Geometry check sheet. Reference: the model listing, model coordinates, mm. Coordinates: 2 decimals unless noted, no trailing zeros. Write each loop counter-clockwise with the first axis right and the second up, starting at its lowest first coordinate (ties: lowest second). Pieces come first, ordered by that corner, then holes. Notation, with made-up numbers: (36, -13.5) -> (80, -13.5) arc R38 cw to (80, 25.5) -> close; hole circle Ø3 at (-1, -25.75). An arc over 180 degrees is marked (long way). Answer as CSV lines item,"result".
```python
from build123d import *

# Parameters (mm, degrees)
SKETCH_1_R      = 11
SKETCH_1_R_2    = 1.5
SKETCH_1_R_3    = 13.5
SKETCH_1_R_4    = 0.5
SKETCH_1_W      = 19.5
SKETCH_1_H      = 19.5
EXTRUDE_1_DEPTH = 3


with BuildPart() as part:
    # 草图1 → 凸台-拉伸1 (new body)
    with BuildSketch(Plane(origin=(0, 0, 0), x_dir=(1, 0, 0), z_dir=(0, 1, 0))):
        with BuildLine():
            Line((10, 0), (136.884360712, 0))
            ThreePointArc((136.884360712, 0), (137.900113715, -0.277140216), (138.634360712, -1.031754163))
            Line((138.634360712, -1.031754163), (139.429147615, -2.468245837))
            ThreePointArc((139.429147615, -2.468245837), (140.163394612, -3.222859784), (141.179147615, -3.5))
            Line((141.179147615, -3.5), (168.820852385, -3.5))
            ThreePointArc((168.820852385, -3.5), (169.836605388, -3.222859784), (170.570852385, -2.468245837))
            Line((170.570852385, -2.468245837), (171.365639288, -1.031754163))
            ThreePointArc((171.365639288, -1.031754163), (172.099886285, -0.277140216), (173.115639288, 0))
            Line((173.115639288, 0), (300, 0))
            ThreePointArc((300, 0), (307.071067812, -2.928932188), (310, -10))
            Line((310, -10), (310, -210))
            ThreePointArc((310, -210), (307.071067812, -217.071067812), (300, -220))
            Line((300, -220), (10, -220))
            ThreePointArc((10, -220), (2.928932188, -217.071067812), (0, -210))
            Line((0, -210), (0, -10))
            ThreePointArc((0, -10), (2.928932188, -2.928932188), (10, 0))
        make_face()
        with Locations(Location((173, -85, 0), (0, 0, 270))):
            Circle(SKETCH_1_R, mode=Mode.SUBTRACT)
        with Locations(Location((190, -66, 0), (0, 0, 270))):
            Circle(SKETCH_1_R, mode=Mode.SUBTRACT)
        with Locations(Location((215, -58, 0), (0, 0, 270))):
            Circle(SKETCH_1_R, mode=Mode.SUBTRACT)
        with Locations(Location((222, -84, 0), (0, 0, 270))):
            Circle(SKETCH_1_R, mode=Mode.SUBTRACT)
        with Locations(Location((247, -84, 0), (0, 0, 270))):
            Circle(SKETCH_1_R, mode=Mode.SUBTRACT)
        with Locations(Location((241, -58, 0), (0, 0, 270))):
            Circle(SKETCH_1_R, mode=Mode.SUBTRACT)
        with Locations(Location((14, -14, 0), (0, 0, 270))):
            Circle(SKETCH_1_R_2, mode=Mode.SUBTRACT)
        with Locations(Location((14, -206, 0), (0, 0, 270))):
            Circle(SKETCH_1_R_2, mode=Mode.SUBTRACT)
        with Locations(Location((296, -206, 0), (0, 0, 270))):
            Circle(SKETCH_1_R_2, mode=Mode.SUBTRACT)
        with Locations(Location((296, -12.28568254, 0), (0, 0, 270))):
            Circle(SKETCH_1_R_2, mode=Mode.SUBTRACT)
        with Locations(Location((198, -90, 0), (0, 0, 270))):
            Circle(SKETCH_1_R, mode=Mode.SUBTRACT)
        with Locations(Location((114, -130, 0), (0, 0, 270))):
            Circle(SKETCH_1_R_3, mode=Mode.SUBTRACT)
        with Locations(Location((190, -130, 0), (0, 0, 270))):
            Circle(SKETCH_1_R_3, mode=Mode.SUBTRACT)
        with Locations(Location((155, -206, 0), (0, 0, 270))):
            Circle(SKETCH_1_R_2, mode=Mode.SUBTRACT)
        with Locations(Location((175, -14, 0), (0, 0, 270))):
            Circle(SKETCH_1_R_2, mode=Mode.SUBTRACT)
        with Locations(Location((145, -138, 0), (0, 0, 270))):
            Circle(SKETCH_1_R, mode=Mode.SUBTRACT)
        with Locations(Location((106, -90, 0), (0, 0, 270))):
            Circle(SKETCH_1_R, mode=Mode.SUBTRACT)
        with Locations(Location((84, -77, 0), (0, 0, 270))):
            Circle(SKETCH_1_R, mode=Mode.SUBTRACT)
        with Locations(Location((58, -80, 0), (0, 0, 270))):
            Circle(SKETCH_1_R, mode=Mode.SUBTRACT)
        with Locations(Location((36, -97, 0), (0, 0, 270))):
            Circle(SKETCH_1_R, mode=Mode.SUBTRACT)
        with Locations(Location((89, -53, 0), (0, 0, 270))):
            Circle(SKETCH_1_R, mode=Mode.SUBTRACT)
        with Locations(Location((266, -66, 0), (0, 0, 270))):
            Circle(SKETCH_1_R, mode=Mode.SUBTRACT)
        with Locations(Location((135, -14, 0), (0, 0, 270))):
            Circle(SKETCH_1_R_2, mode=Mode.SUBTRACT)
        with Locations(Location((296, -110, 0), (0, 0, 270))):
            Circle(SKETCH_1_R_2, mode=Mode.SUBTRACT)
        with Locations(Location((14, -110, 0), (0, 0, 270))):
            Circle(SKETCH_1_R_2, mode=Mode.SUBTRACT)
        with Locations(Location((152, -16, 0), (0, 0, 270))):
            Circle(SKETCH_1_R_4, mode=Mode.SUBTRACT)
        with Locations((38, -24)):
            Rectangle(SKETCH_1_W, SKETCH_1_H, mode=Mode.SUBTRACT)
        with Locations((62, -24)):
            Rectangle(SKETCH_1_W, SKETCH_1_H, mode=Mode.SUBTRACT)
        with Locations((86, -24)):
            Rectangle(SKETCH_1_W, SKETCH_1_H, mode=Mode.SUBTRACT)
        with Locations((110, -24)):
            Rectangle(SKETCH_1_W, SKETCH_1_H, mode=Mode.SUBTRACT)
        with Locations((198, -24)):
            Rectangle(SKETCH_1_W, SKETCH_1_H, mode=Mode.SUBTRACT)
        with Locations((222, -24)):
            Rectangle(SKETCH_1_W, SKETCH_1_H, mode=Mode.SUBTRACT)
        with Locations((246, -24)):
            Rectangle(SKETCH_1_W, SKETCH_1_H, mode=Mode.SUBTRACT)
        with Locations((270, -24)):
            Rectangle(SKETCH_1_W, SKETCH_1_H, mode=Mode.SUBTRACT)
    extrude(amount=EXTRUDE_1_DEPTH)


solid = part.part
```
Item 1: Thickness scan on probe 1 along Z at (x, y) = (65.5, 2.65); probe 2 along Z at (x, y) = (152, 0.95); probe 3 along X at (y, z) = (1.5, 121.5). Record the ranges inside material, lowest first.
Responses:
probe 1,"z = 0 to 14.25, 33.75 to 71.95, 88.05 to 220"
probe 2,"z = 3.5 to 15.5, 16.5 to 129.51, 146.49 to 220"
probe 3,"x = 0 to 103.51, 124.49 to 179.51, 200.49 to 310"
Item 2: Depth check by flat-ended pin: pin 1 Ø13 at (x, z) = (89, 53) entering from -Y. Enter the tip coordinate at first touch or a pass-through.
Responses:
pin 1,"passes through"
Item 3: Cross-section at B-B, the plane y = 1.15. Count the separate pieces of the cut face and the enclosed holes in it, plus the area to 3 significant figures.
Responses:
separate pieces,"1"
enclosed holes,"34"
area,"58,400 mm2"
Item 4: Release check for a two-part mould opening along X. For faces 1 (the cylindrical face through (3.01, 1.48, 217.15)), 2 (the flat face through (157, 0, 108)), 3 (the cylindrical face through (257.906, 1.479, 82.568)) record: +X half, -X half, draft (parallel to the pull), parting line (faces both ways), or undercut.
Responses:
face 1,"-X half"
face 2,"draft"
face 3,"undercut"
Item 5: Cross-section at D-D, the plane x = 89. Record the cut outline in (y, z), plus the area to 3 significant figures.
Responses:
outline,"(0, 0) -> (3, 0) -> (3, 14.25) -> (0, 14.25) -> close; (0, 33.75) -> (3, 33.75) -> (3, 42) -> (0, 42) -> close; (0, 64) -> (3, 64) -> (3, 67.2) -> (0, 67.2) -> close; (0, 86.8) -> (3, 86.8) -> (3, 220) -> (0, 220) -> close"
area,"477 mm2"
Item 6: Cross-section at C-C, the plane z = 134. Record the cut outline in (x, y).
Responses:
outline,"(0, 0) -> (101.11, 0) -> (101.11, 3) -> (0, 3) -> close; (126.89, 0) -> (134.75, 0) -> (134.75, 3) -> (126.89, 3) -> close; (155.25, 0) -> (177.11, 0) -> (177.11, 3) -> (155.25, 3) -> close; (202.89, 0) -> (310, 0) -> (310, 3) -> (202.89, 3) -> close"
Item 7: Cross-section at A-A, the plane x = 36. Record the cut outline in (y, z), plus the area to 4 significant figures.
Responses:
outline,"(0, 0) -> (3, 0) -> (3, 14.25) -> (0, 14.25) -> close; (0, 33.75) -> (3, 33.75) -> (3, 86) -> (0, 86) -> close; (0, 108) -> (3, 108) -> (3, 220) -> (0, 220) -> close"
area,"535.5 mm2"
